from build123d import *

# Parameters (mm, degrees)
SKETCH_1_W          = 109
SKETCH_1_H          = 31
EXTRUDE_1_DEPTH     = 2
SKETCH_2_W          = 2.5
SKETCH_2_H          = 8
EXTRUDE_2_DEPTH     = 2
SKETCH_3_W          = 15
SKETCH_3_H          = 2.5
EXTRUDE_3_DEPTH     = 2
CUT_EXTRUDE_1_DEPTH = 117.44097217
CUT_EXTRUDE_2_DEPTH = 117.44097217


with BuildPart() as part:
    # 草图1 → 凸台-拉伸1 (new body)
    with BuildSketch(Plane.XY):
        with Locations((54.5, 15.5)):
            Rectangle(SKETCH_1_W, SKETCH_1_H)
        Polygon((23.3, 3.5), (28.3, 3.5), (29.3, 2.5), (59.3, 2.5), (60.3, 3.5), (65.3, 3.5), (66.3, 2.5), (77.3, 2.5), (78.3, 3.5), (83.3, 3.5), (84.3, 2.5), (102.6, 2.5), (102.6, 7.5), (103.6, 8.5), (103.6, 20.1), (85.8, 20.1), (84.8, 19.1), (79.8, 19.1), (78.8, 20.1), (54.3, 20.1), (53.3, 19.1), (48.3, 19.1), (47.3, 20.1), (29.8, 20.1), (28.8, 19.1), (23.8, 19.1), (22.8, 20.1), (5.3, 20.1), (5.3, 13.5), (6.3, 12.5), (6.3, 7.5), (5.3, 6.5), (5.3, 2.5), (22.3, 2.5), align=None, mode=Mode.SUBTRACT)
    extrude(amount=EXTRUDE_1_DEPTH)

    # 草图2 → 凸台-拉伸2 (add)
    with BuildSketch(Plane.XY.offset(2)):
        with Locations((-1.25, 22)):
            Rectangle(SKETCH_2_W, SKETCH_2_H)
        with Locations((-1.25, 9)):
            Rectangle(SKETCH_2_W, SKETCH_2_H)
        with Locations((110.25, 9)):
            Rectangle(SKETCH_2_W, SKETCH_2_H)
        with Locations((110.25, 22)):
            Rectangle(SKETCH_2_W, SKETCH_2_H)
    extrude(amount=-EXTRUDE_2_DEPTH)

    # 草图3 → 凸台-拉伸3 (add)
    with BuildSketch(Plane.XY.offset(2)):
        with Locations((17.5, 32.25)):
            Rectangle(SKETCH_3_W, SKETCH_3_H)
        with Locations((54.5, 32.25)):
            Rectangle(SKETCH_3_W, SKETCH_3_H)
        with Locations((91.5, 32.25)):
            Rectangle(SKETCH_3_W, SKETCH_3_H)
        with Locations((91.5, -1.25)):
            Rectangle(SKETCH_3_W, SKETCH_3_H)
        with Locations((54.5, -1.25)):
            Rectangle(SKETCH_3_W, SKETCH_3_H)
        with Locations((17.5, -1.25)):
            Rectangle(SKETCH_3_W, SKETCH_3_H)
    extrude(amount=-EXTRUDE_3_DEPTH)

    # 草图4 → 切除-拉伸1 (cut, through all)
    with BuildSketch(Plane.XY.offset(2)):
        with BuildLine():
            Line((8, 31), (10, 31))
            ThreePointArc((10, 31), (9, 30), (8, 31))
        make_face()
        with BuildLine():
            Line((27, 31), (25, 31))
            ThreePointArc((25, 31), (26, 30), (27, 31))
        make_face()
        with BuildLine():
            Line((45, 31), (47, 31))
            ThreePointArc((47, 31), (46, 30), (45, 31))
        make_face()
        with BuildLine():
            Line((64, 31), (62, 31))
            ThreePointArc((62, 31), (63, 30), (64, 31))
        make_face()
        with BuildLine():
            Line((82, 31), (84, 31))
            ThreePointArc((84, 31), (83, 30), (82, 31))
        make_face()
        with BuildLine():
            Line((101, 31), (99, 31))
            ThreePointArc((99, 31), (100, 30), (101, 31))
        make_face()
        with BuildLine():
            Line((101, 0), (99, 0))
            ThreePointArc((99, 0), (100, 1), (101, 0))
        make_face()
        with BuildLine():
            Line((82, 0), (84, 0))
            ThreePointArc((84, 0), (83, 1), (82, 0))
        make_face()
        with BuildLine():
            Line((64, 0), (62, 0))
            ThreePointArc((62, 0), (63, 1), (64, 0))
        make_face()
        with BuildLine():
            Line((45, 0), (47, 0))
            ThreePointArc((47, 0), (46, 1), (45, 0))
        make_face()
        with BuildLine():
            Line((27, 0), (25, 0))
            ThreePointArc((25, 0), (26, 1), (27, 0))
        make_face()
        with BuildLine():
            Line((8, 0), (10, 0))
            ThreePointArc((10, 0), (9, 1), (8, 0))
        make_face()
    extrude(amount=-CUT_EXTRUDE_1_DEPTH, mode=Mode.SUBTRACT)

    # 草图5 → 切除-拉伸2 (cut, through all)
    with BuildSketch(Plane.XY.offset(2)):
        with BuildLine():
            Line((6, 27.5), (31, 27.5))
            ThreePointArc((31, 27.5), (33, 25.5), (31, 23.5))
            Line((31, 23.5), (6, 23.5))
            ThreePointArc((6, 23.5), (4, 25.5), (6, 27.5))
        make_face()
        with BuildLine():
            Line((42, 27.5), (67, 27.5))
            ThreePointArc((67, 27.5), (69, 25.5), (67, 23.5))
            Line((67, 23.5), (42, 23.5))
            ThreePointArc((42, 23.5), (40, 25.5), (42, 27.5))
        make_face()
        with BuildLine():
            Line((78, 27.5), (103, 27.5))
            ThreePointArc((103, 27.5), (105, 25.5), (103, 23.5))
            Line((103, 23.5), (78, 23.5))
            ThreePointArc((78, 23.5), (76, 25.5), (78, 27.5))
        make_face()
    extrude(amount=-CUT_EXTRUDE_2_DEPTH, mode=Mode.SUBTRACT)


solid = part.part
Part model, mm, in its own coordinate system. A direction names the side the tool comes from. Round coordinates to 2 decimals unless told otherwise and drop trailing zeros. Order: outer loops, then holes, each group sorted by start corner. A loop starts at its lowest first (then second) coordinate and runs counter-clockwise, first axis right, second up. Notation, with made-up numbers: (14, 34.25) -> (48, 34.25) arc R24 cw to (48, 56.25) -> close; hole circle Ø7 at (12.25, 78.25). An arc over 180 degrees is marked (long way). Put each result on its own line as item: value.
Q1. Band-saw the part on A-A (x = 46). Give the cut face in (y, z), and give its area (3 significant figures).
From the geometry:
outline: (1, 0) -> (2.5, 0) -> (2.5, 2) -> (1, 2) -> close; (20.1, 0) -> (23.5, 0) -> (23.5, 2) -> (20.1, 2) -> close; (27.5, 0) -> (30, 0) -> (30, 2) -> (27.5, 2) -> close
area: 14.8 mm2
Q2. Band-saw the part on C-C (x = 98). Give the cut face in (y, z), and give its area (3 significant figures).
From the geometry:
outline: (-2.5, 0) -> (2.5, 0) -> (2.5, 2) -> (-2.5, 2) -> close; (20.1, 0) -> (23.5, 0) -> (23.5, 2) -> (20.1, 2) -> close; (27.5, 0) -> (33.5, 0) -> (33.5, 2) -> (27.5, 2) -> close
area: 28.8 mm2
Q3. Pin check, flat tips, straight feed: pin 1 Ø1 at (x, z) = (70, 1) entering from -Y; pin 2 Ø0.6 at (y, z) = (16.5, 1) entering from +X; pin 3 Ø1 at (x, z) = (-1.5, 1.5) entering from +Y. Stop position of each tip, or through.
From the geometry:
pin 1: stops at y = 0
pin 2: stops at x = 109
pin 3: stops at y = 26
Q4. Band-saw the part on D-D (z = 0.8). State how many separate pieces and enclosed holes the cut face has, and give its area (3 significant figures).
From the geometry:
separate pieces: 1
enclosed holes: 4
area: 1,640 mm2
Q5. Tool access for faces 1 (the face through (110, 26, 1)), 2 (the face through (84, -1, 1)), 3 (the face through (10, 32, 1)), 4 (the face through (109, 2, 1)), 5 (the face through (25, 32, 1)): list every direction of +Z, -Z, +X, -X, +Y, -Y with a clear straight run to the whole face (end or side of a thin tool).
From the geometry:
face 1: +Z, -Z, +X, +Y
face 2: +Z, -Z, -Y
face 3: +Z, -Z, -X, +Y
face 4: +Z, -Z, +X, -Y
face 5: +Z, -Z, +Y
Q6. Band-saw the part on B-B (y = 11). Give the cut face in (x, z), and give its area (3 significant figures).
From the geometry:
outline: (-2.5, 0) -> (6.3, 0) -> (6.3, 2) -> (-2.5, 2) -> close; (103.6, 0) -> (111.5, 0) -> (111.5, 2) -> (103.6, 2) -> close
area: 33.4 mm2
Q7. Wall check: line 1 (Y direction, x = 91.5, z = 0.7); line 2 (Y direction, x = 83, z = 0.75); line 3 (Y direction, x = 34.5, z = 0.9). Give the ranges that are in metal, low to high. Write a range as [from, to].
From the geometry:
line 1: y = [-2.5, 2.5], [20.1, 23.5], [27.5, 33.5]
line 2: y = [1, 3.5], [19.1, 23.5], [27.5, 30]
line 3: y = [0, 2.5], [20.1, 31]
Q8. Pull direction X, two halves, no side cores. Call faces 6 (the face through (95, 20.1, 1)), 7 (the face through (105, 31, 1)), 8 (the face through (-2.5, 22, 1)): pulls with the +X half, pulls with the -X half, needs draft (parallel to the pull), parting line crosses it, or undercut.
From the geometry:
face 6: undercut
face 7: needs draft
face 8: pulls with the -X half
